Geometry: final body of the model. Coordinates: model frame, mm. Face numbers are marked on the shaded views. A direction names the side the tool comes from. Round coordinates to 2 decimals unless told otherwise and drop trailing zeros. Loops run counter-clockwise (first coordinate to the right, second up) from the corner with the lowest first, then second, coordinate; pieces in that order, holes last. Notation, with made-up numbers: (57, 40) - (109, 40) arc R12 cw to (109, 53) - close; hole circle Ø1 at (1.25, -39.5). An arc over 180 degrees is marked (long way). Answer in a Markdown table with one row per item. Add a question column.
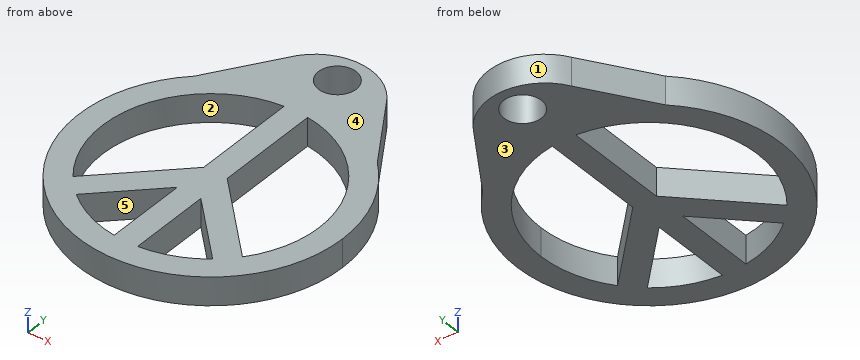
from build123d import *

# Parameters (mm, degrees)
F1_R     = 2
F2_DEPTH = 3


with BuildPart() as f2:
    # F1 (on Top) → F2 (new body)
    with BuildSketch(Plane.XY):
        with BuildLine():
            ThreePointArc((-9.7114153746, 10.0840672063), (-5.4790594428, -12.8833189676), (14, 0))
            ThreePointArc((14, 0), (12.8833189676, 5.4790594428), (9.7114153746, 10.0840672063))
            ThreePointArc((9.7114153746, 10.0840672063), (7.8963049332, 11.5606387541), (5.8606261419, 12.7142857143))
            ThreePointArc((5.8606261419, 12.7142857143), (0, 14), (-5.8606261419, 12.7142857143))
            ThreePointArc((-5.8606261419, 12.7142857143), (-7.8963049332, 11.5606387541), (-9.7114153746, 10.0840672063))
        make_face()
        with BuildLine():
            ThreePointArc((1.25, 11.4318633652), (8.5622718948, 7.6770762664), (11.5, 0))
            ThreePointArc((11.5, 0), (10.8590955773, -3.7855043577), (9.0078185666, -7.1490701963))
            ThreePointArc((9.0078185666, -7.1490701963), (8.1773610714, -8.0858373659), (7.25, -8.9267855357))
            ThreePointArc((7.25, -8.9267855357), (4.4307283524, -10.6121932826), (1.25, -11.4318633652))
            ThreePointArc((1.25, -11.4318633652), (0, -11.5), (-1.25, -11.4318633652))
            ThreePointArc((-1.25, -11.4318633652), (-4.4307283524, -10.6121932826), (-7.25, -8.9267855357))
            ThreePointArc((-7.25, -8.9267855357), (-8.1773610714, -8.0858373659), (-9.0078185666, -7.1490701963))
            ThreePointArc((-9.0078185666, -7.1490701963), (-10.6121856109, 4.4307467271), (-1.25, 11.4318633652))
            ThreePointArc((-1.25, 11.4318633652), (0, 11.5), (1.25, 11.4318633652))
        make_face(mode=Mode.SUBTRACT)
        with BuildLine():
            ThreePointArc((5.8606261419, 12.7142857143), (7.8963049332, 11.5606387541), (9.7114153746, 10.0840672063))
            Line((9.7114153746, 10.0840672063), (5.1961524227, 17))
            ThreePointArc((5.1961524227, 17), (5.9291588604, 14.9192797226), (5.8606261419, 12.7142857143))
        make_face()
        with BuildLine():
            Line((-5.1961524227, 17), (-9.7114153746, 10.0840672063))
            ThreePointArc((-9.7114153746, 10.0840672063), (-7.8963049332, 11.5606387541), (-5.8606261419, 12.7142857143))
            ThreePointArc((-5.8606261419, 12.7142857143), (-5.9291588604, 14.9192797226), (-5.1961524227, 17))
        make_face()
        with BuildLine():
            ThreePointArc((-5.8606261419, 12.7142857143), (0, 14), (5.8606261419, 12.7142857143))
            ThreePointArc((5.8606261419, 12.7142857143), (5.9291588604, 14.9192797226), (5.1961524227, 17))
            ThreePointArc((5.1961524227, 17), (0, 20), (-5.1961524227, 17))
            ThreePointArc((-5.1961524227, 17), (-5.9291588604, 14.9192797226), (-5.8606261419, 12.7142857143))
        make_face()
        with Locations((0, 17)):
            Circle(F1_R, mode=Mode.SUBTRACT)
        with BuildLine():
            Line((1.25, 0.6087483703), (1.25, 11.4318633652))
            ThreePointArc((1.25, 11.4318633652), (0, 11.5), (-1.25, 11.4318633652))
            Line((-1.25, 11.4318633652), (-1.25, 0.6087483703))
            Line((-1.25, 0.6087483703), (-9.0078185666, -7.1490701963))
            ThreePointArc((-9.0078185666, -7.1490701963), (-8.1773610714, -8.0858373659), (-7.25, -8.9267855357))
            Line((-7.25, -8.9267855357), (-1.25, -2.9267855357))
            Line((-1.25, -2.9267855357), (-1.25, -11.4318633652))
            ThreePointArc((-1.25, -11.4318633652), (0, -11.5), (1.25, -11.4318633652))
            Line((1.25, -11.4318633652), (1.25, -2.9267855357))
            Line((1.25, -2.9267855357), (7.25, -8.9267855357))
            ThreePointArc((7.25, -8.9267855357), (8.1773610714, -8.0858373659), (9.0078185666, -7.1490701963))
            Line((9.0078185666, -7.1490701963), (1.25, 0.6087483703))
        make_face()
    extrude(amount=F2_DEPTH)


solid = f2.part
1) Material intervals for line 1 along Y through (x, z) = (0, 0.9); line 2 along X through (y, z) = (-4, 1.5); line 3 along X through (y, z) = (-1, 0.65), sorted ascending. Write a range as from..to.
2) Section B-B, the plane z = 1.4. Return the cut outline in (x, y), and give its area (3 significant figures).
3) Contact query for flat-ended pins moving along their axis: pin 1 Ø8 at (x, y) = (-10, 10) entering from -Z; pin 2 Ø1.5 at (y, z) = (6, 1.5) entering from +X; pin 3 Ø1.5 at (y, z) = (-6.5, 2) entering from +X; pin 4 Ø0.9 at (y, z) = (-7, 1) entering from -X. Output: stop coordinate, or through.
4) Section C-C, the plane y = -1.5. Return the cut outline in (x, z), and give its area (3 significant figures).
5) Pull-direction query (Y, two-part tool) for the marked faces 1, 2 and 3; classes: pulls with the +Y half, pulls with the -Y half, needs draft (parallel to the pull), parting line crosses it, or undercut.
6) Section A-A, the plane x = 0. Return the cut outline in (y, z), and give its area (3 significant figures).
7) Section D-D, the plane y = -5. Return the cut outline in (x, z).
8) Reachability of the marked faces 4 and 5 from +Z, -Z, +X, -X, +Y, -Y: full face, straight path, thin tool, end or side. Return the list, or none.
Evaluation:
| question | item | result |
|---|---|---|
| 1 | line 1 | y = -14..15, 19..20 |
| 1 | line 2 | x = -13.42..-10.78, -5.86..-2.32, -1.25..1.25, 2.32..5.86, 10.78..13.42 |
| 1 | line 3 | x = -13.96..-11.46, -2.86..2.86, 11.46..13.96 |
| 2 | outline | (-9.71, 10.08) arc R14 ccw (long way) to (9.71, 10.08) - (5.2, 17) arc R6 ccw to (-5.2, 17) - close; hole (-9.01, -7.15) - (-1.25, 0.61) - (-1.25, 11.43) arc R11.5 ccw to start; hole (-7.25, -8.93) arc R11.5 ccw to (-1.25, -11.43) - (-1.25, -2.93) - close; hole circle Ø4 at (0, 17); hole (1.25, -11.43) arc R11.5 ccw to (7.25, -8.93) - (1.25, -2.93) - close; hole (1.25, 0.61) - (9.01, -7.15) arc R11.5 ccw to (1.25, 11.43) - close |
| 2 | area | 367 mm² |
| 3 | pin 1 | stops at z = 0 |
| 3 | pin 2 | stops at x = 12.98 |
| 3 | pin 3 | stops at x = 12.76 |
| 3 | pin 4 | stops at x = -12.37 |
| 4 | outline | (-13.92, 0) - (-11.4, 0) - (-11.4, 3) - (-13.92, 3) - close; (-3.36, 0) - (3.36, 0) - (3.36, 3) - (-3.36, 3) - close; (11.4, 0) - (13.92, 0) - (13.92, 3) - (11.4, 3) - close |
| 4 | area | 35.3 mm² |
| 5 | face 1 | pulls with the +Y half |
| 5 | face 2 | undercut |
| 5 | face 3 | needs draft |
| 6 | outline | (-14, 0) - (15, 0) - (15, 3) - (-14, 3) - close; (19, 0) - (20, 0) - (20, 3) - (19, 3) - close |
| 6 | area | 90.0 mm² |
| 7 | outline | (-13.08, 0) - (-10.36, 0) - (-10.36, 3) - (-13.08, 3) - close; (-6.86, 0) - (-3.32, 0) - (-3.32, 3) - (-6.86, 3) - close; (-1.25, 0) - (1.25, 0) - (1.25, 3) - (-1.25, 3) - close; (3.32, 0) - (6.86, 0) - (6.86, 3) - (3.32, 3) - close; (10.36, 0) - (13.08, 0) - (13.08, 3) - (10.36, 3) - close |
| 8 | face 4 | +Z, +X, -X, +Y, -Y |
| 8 | face 5 | +Z, -Z |
